For this review, use the dimensioned drawing (mm, ordinates from the lowest corner) and the shaded views. A direction names the side the tool comes from. Round coordinates to 2 decimals unless told otherwise and drop trailing zeros. Loops run counter-clockwise (first coordinate to the right, second up) from the corner with the lowest first, then second, coordinate; pieces in that order, holes last. Notation, with made-up numbers: M -35.5,58.5 L -30.5,58.5 A29 ccw -30.5,89.5 Z; hole C -32.5,69 d7. An arc over 180 degrees is marked long. Answer as a JSON object with one key per item and string values. Group by question number.
Item 1: Tool access review of the marked faces 1, 2, 3 and 4: name each direction out of +Z, -Z, +X, -X, +Y, -Y from which nothing blocks a thin tool from reaching the whole face with its end or side.
Item 2: Insertion check: P1, Ø1, axis at x = 23.5, y = 6.5, coming from the +Z side; P2, Ø3, axis at y = 7.5, z = 8, coming from the +X side; P3, Ø1.5, axis at y = 4.5, z = 11.5, coming from the +X side. Each pin has a flat end and moves straight along its axis. Give the tip position at first contact, or say it passes through.
Item 3: The part is to be moulded in two halves that separate along X. For the marked faces 5, 6 and 7, say which applies: +X half, -X half, draft (parallel to the pull), parting line (faces both ways), or undercut.
Item 4: Consider section B-B (y = 19). Give the boundary of the cut face in (x, z).
Item 5: Consider section C-C (z = 8). Give the boundary of the cut face in (x, y), and give its area (3 significant figures).
Item 6: Consider section A-A (x = 21.5). Give the boundary of the cut face in (y, z).
Item 7: Consider section D-D (x = 35.5). Give the boundary of the cut face in (y, z), and give its area (3 significant figures).
Item 8: To check wall thickness, follow line 1 (X direction, y = 18.75, z = 3.5); line 2 (Y direction, x = 21.5, z = 5.25); line 3 (Y direction, x = 21.5, z = 2.5). State the ranges of each line that lie inside material, in increasing order.
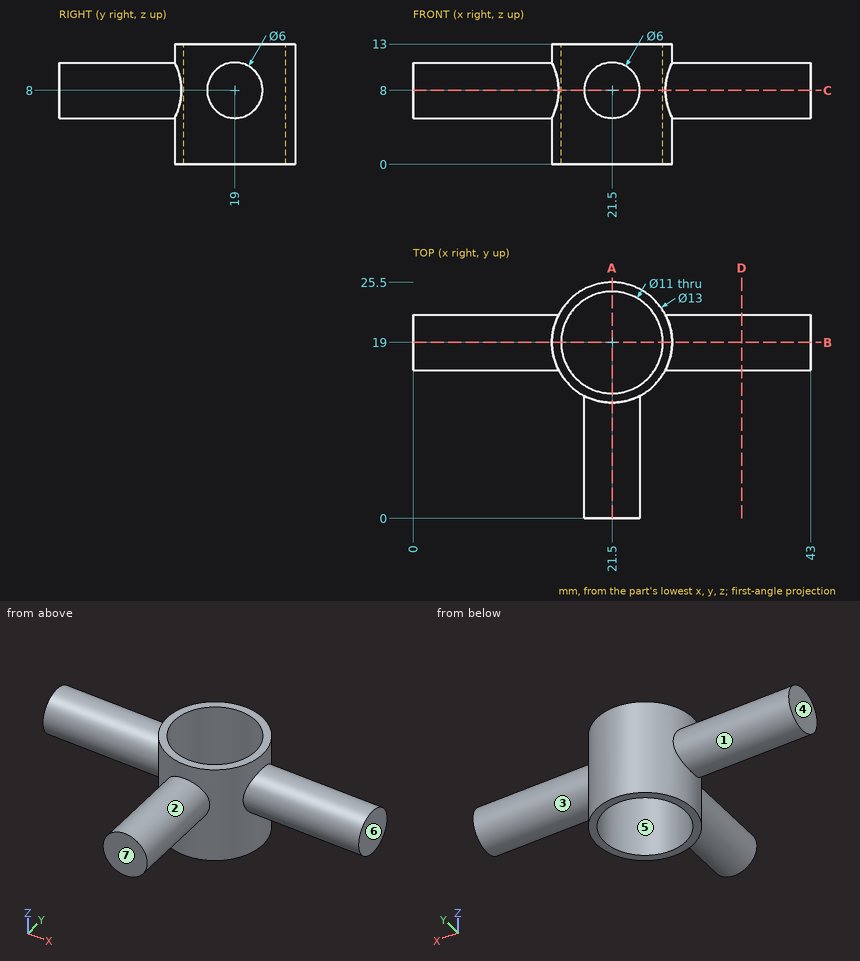
Geometry results:
{
 "1": {"face 1": "-X", "face 2": "-Y", "face 3": "+X", "face 4": "+Z, -Z, -X, +Y, -Y"},
 "2": {"P1": "stops at z = 10.6", "P2": "stops at x = 24.5", "P3": "stops at x = 22.7"},
 "3": {"face 5": "undercut", "face 6": "+X half", "face 7": "draft"},
 "4": {"outline": "M 0,5 L 15,5 L 15,0 L 16,0 L 16,13 L 15,13 L 15,11 L 0,11 Z; M 27,0 L 28,0 L 28,5 L 43,5 L 43,11 L 28,11 L 28,13 L 27,13 Z"},
 "5": {"outline": "M 0,16 L 15.73,16 A6.5 ccw 18.5,13.23 L 18.5,0 L 24.5,0 L 24.5,13.23 A6.5 ccw 27.27,16 L 43,16 L 43,22 L 27.27,22 A6.5 ccw 15.73,22 L 0,22 Z; hole C 21.5,19 d11", "area": "297 mm^2"},
 "6": {"outline": "M 0,5 L 12.5,5 L 12.5,0 L 13.5,0 L 13.5,13 L 12.5,13 L 12.5,11 L 0,11 Z; M 24.5,0 L 25.5,0 L 25.5,13 L 24.5,13 Z"},
 "7": {"outline": "C 19,8 d6", "area": "28.3 mm^2"},
 "8": {"line 1": "x = 15 to 16.01, 26.99 to 28", "line 2": "y = 0 to 13.5, 24.5 to 25.5", "line 3": "y = 12.5 to 13.5, 24.5 to 25.5"}
}
